```python
from build123d import *

# Parameters (mm, degrees)
F0_W     = 60.96
F0_H     = 38.1
F1_DEPTH = 10.16
F2_W     = 19.05
F2_H     = 38.1
F3_DEPTH = 17.78
F4_W     = 19.05
F4_H     = 10.16
F5_DEPTH = 8.89
F6_R     = 1.27


with BuildPart() as f1:
    # F0 (on Front) → F1 (new body)
    with BuildSketch(Plane.XZ):
        Rectangle(F0_W, F0_H)
    extrude(amount=F1_DEPTH)

    # F2 (on face) → F3 (join)
    with BuildSketch(Plane.XZ.offset(10.16)):
        with Locations((20.955, 0)):
            Rectangle(F2_W, F2_H)
    extrude(amount=F3_DEPTH)

    # F4 (on face) → F5 (join)
    with BuildSketch(Plane.XZ.offset(10.16)):
        with Locations((1.905, 13.97)):
            Rectangle(F4_W, F4_H)
        with Locations((1.905, -13.97)):
            Rectangle(F4_W, F4_H)
    extrude(amount=F5_DEPTH)

    # F6
    f6_edges = [f1.edges().sort_by_distance(p)[0] for p in [
        (-30.48, -5.08, 19.05),
        (-30.48, -5.08, -19.05),
        (-7.62, -14.605, 19.05),
        (-7.62, -14.605, 8.89),
        (-7.62, -14.605, -8.89),
        (-7.62, -14.605, -19.05),
        (11.43, -23.495, -19.05),
        (11.43, -23.495, 19.05),
        (30.48, -13.97, 19.05),
        (30.48, -13.97, -19.05),
        (11.43, -14.605, -8.89),
        (11.43, -14.605, 8.89),
    ]]
    fillet(f6_edges, radius=F6_R)


solid = f1.part
```
CAD build for the part. Positions are in the model's coordinates, mm. A direction names the side the tool comes from. Coordinates: 2 decimals unless noted, no trailing zeros. Loops run counter-clockwise (first coordinate to the right, second up) from the corner with the lowest first, then second, coordinate; pieces in that order, holes last. Notation, with made-up numbers: (-35.75, 68) - (-0.75, 68) arc R27 ccw to (-0.75, 106) - close; hole circle Ø6 at (58, 44). An arc over 180 degrees is marked (long way). Return JSON: item names as keys, results as strings.
1. Band-saw the part on C-C (x = -24). Give the cut face in (y, z).
Result:
{"outline": "(-10.16, -19.05) - (0, -19.05) - (0, 19.05) - (-10.16, 19.05) - close"}
2. Band-saw the part on D-D (y = -12). Give the cut face in (x, z).
Result:
{"outline": "(-7.62, -17.78) arc R1.27 ccw to (-6.35, -19.05) - (29.21, -19.05) arc R1.27 ccw to (30.48, -17.78) - (30.48, 17.78) arc R1.27 ccw to (29.21, 19.05) - (-6.35, 19.05) arc R1.27 ccw to (-7.62, 17.78) - (-7.62, 10.16) arc R1.27 ccw to (-6.35, 8.89) - (10.16, 8.89) arc R1.27 cw to (11.43, 7.62) - (11.43, -7.62) arc R1.27 cw to (10.16, -8.89) - (-6.35, -8.89) arc R1.27 ccw to (-7.62, -10.16) - close"}
3. Band-saw the part on B-B (y = -24). Give the cut face in (x, z).
Result:
{"outline": "(11.43, -17.78) arc R1.27 ccw to (12.7, -19.05) - (29.21, -19.05) arc R1.27 ccw to (30.48, -17.78) - (30.48, 17.78) arc R1.27 ccw to (29.21, 19.05) - (12.7, 19.05) arc R1.27 ccw to (11.43, 17.78) - close"}
4. Drop flat-ended pins along their axis: pin 1 (1.5 mm diameter, centred on y = -13.5, z = -12.5, fed in from -X); pin 2 (5.5 mm diameter, centred on x = 1, z = 15, fed in from -Y); pin 3 (6 mm diameter, centred on x = -12.5, y = -21.5, fed in from +Z); pin 4 (6 mm diameter, centred on y = -12.5, z = 13.5, fed in from -X). Give the stop position or say it passes through.
Result:
{"pin 1": "stops at x = -7.62", "pin 2": "stops at y = -19.05", "pin 3": "passes through", "pin 4": "stops at x = -30.48"}
5. Probe L1, parallel to Z at x = 8.5, y = -12.5; L2, parallel to Y at x = 11, z = -16; L3, parallel to Y at x = -23, z = 7. List the from-to ranges inside material, lowest first. Write a range as from..to.
Result:
{"L1": "z = -19.05..-8.89, 8.89..19.05", "L2": "y = -19.05..0", "L3": "y = -10.16..0"}
6. Band-saw the part on A-A (z = 15.5). Give the cut face in (x, y).
Result:
{"outline": "(-30.48, -10.16) - (-7.62, -10.16) - (-7.62, -19.05) - (11.43, -19.05) - (11.43, -27.94) - (30.48, -27.94) - (30.48, 0) - (-30.48, 0) - close"}
7. 3-axis set-ups, long thin cutter, end or side, ignore diameter. For faces 4 (the flat face through (-7.62, -15, 14)), 5 (the flat face through (-14, -10.16, 0)), 6 (the cylindrical face through (11.792, -23.557, -18.668)): which of +Z, -Z, +X, -X, +Y, -Y reach the whole face in a straight line?
Result:
{"face 4": "+Z, -Z, -X, -Y", "face 5": "-X, -Y", "face 6": "-Z, -X, -Y"}
8. Mould opens along Z. For faces 1 (the flat face through (11.43, -21, 0)), 2 (the cylindrical face through (30.098, -13.774, 18.688)), 3 (the flat face through (2, -19.05, 13)) say: released by +Z, released by -Z, zero draft, split by the parting line, or undercut.
Result:
{"face 1": "undercut", "face 2": "released by +Z", "face 3": "zero draft"}
